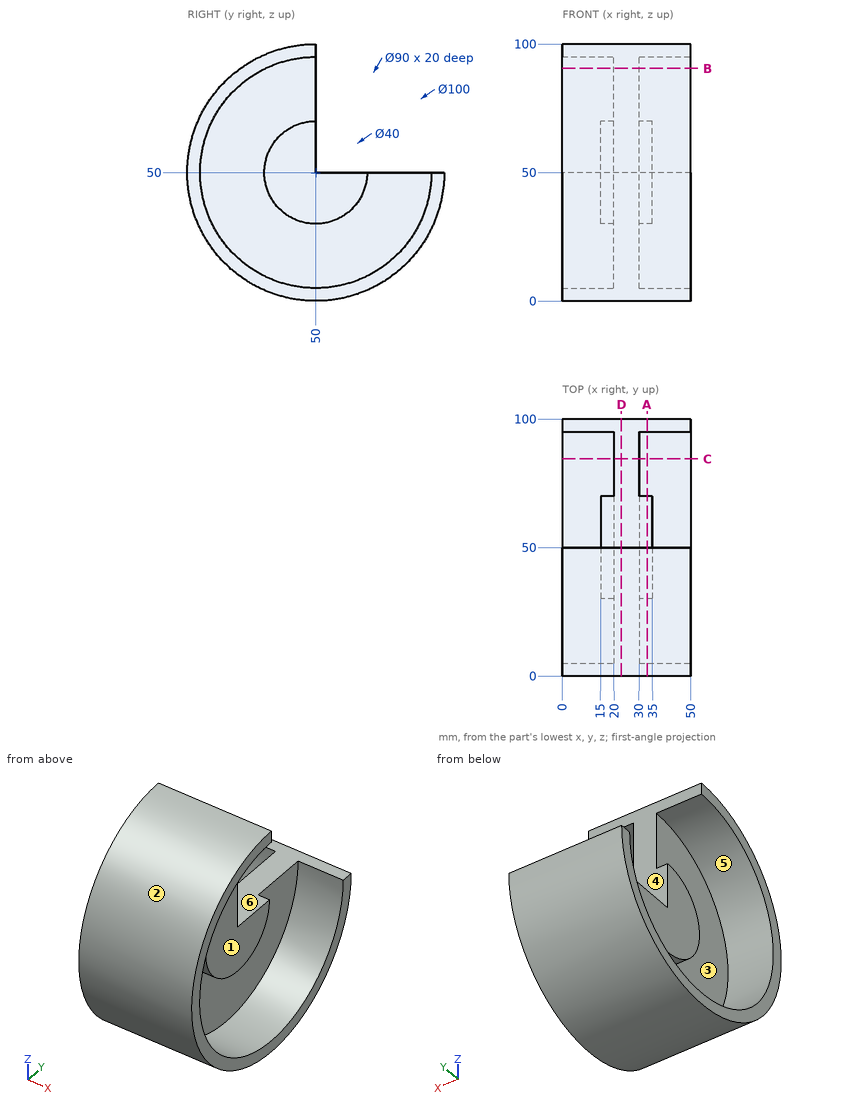
For this review, use the dimensioned drawing (mm, ordinates from the lowest corner) and the shaded views. A direction names the side the tool comes from. Give positions to 0.01 mm unless a question says otherwise; leave off trailing zeros. Loops run counter-clockwise (first coordinate to the right, second up) from the corner with the lowest first, then second, coordinate; pieces in that order, holes last. Notation, with made-up numbers: (-11, 83.5) -> (-5, 83.5) arc R22 ccw to (-5, 99.5) -> close; hole circle Ø7 at (3.5, -12). An arc over 180 degrees is marked (long way). One line per question, with ' | ' between items. Start each with the question number.
(1) Insertion check: P1, Ø1, axis at x = 20, y = 63, coming from the +Z side; P2, Ø10, axis at x = 29, z = 44.5, coming from the +Y side; P3, Ø20, axis at y = 54.5, z = 46.5, coming from the -X side. Each pin has a flat end and moves straight along its axis. Give the tip position at first contact, or say it passes through.
(2) Draft analysis for pull direction Y (two halves, no side actions). For the marked faces 4, 5 and 6, state which applies: +Y half, -Y half, draft (parallel to the pull), parting line (faces both ways), or undercut.
(3) We need section B-B (z = 90.5). State the section outline as (x, y) points, and give its area (3 significant figures).
(4) For the marked faces 1, 2 and 3, list the 3-axis set-ups (+Z, -Z, +X, -X, +Y, -Y) from which the entire face can be reached by the end or side of a thin tool; tool diameter is ignored.
(5) We need section C-C (y = 84.5). State the section outline as (x, z) points, and give its area (3 significant figures).
(6) We need section A-A (x = 33). State the section outline as (y, z) points.
(7) We need section D-D (x = 23). State the section outline as (y, z) points.
(8) For line 1 (X direction, y = 45, z = 82); line 2 (Y direction, x = 4.5, z = 13); line 3 (Y direction, x = 41, z = 16.5), list the stretches that pass through material, from the lowest coordinate up.
The answers:
1) P1: stops at z = 50 | P2: stops at y = 100 | P3: stops at x = 15
2) face 4: +Y half | face 5: undercut | face 6: draft
3) outline: (0, 20.68) -> (50, 20.68) -> (50, 30.38) -> (30, 30.38) -> (30, 50) -> (20, 50) -> (20, 30.38) -> (0, 30.38) -> close | area: 681 mm^2
4) face 1: +X | face 2: +X, -X | face 3: -X
5) outline: (0, 13.81) -> (50, 13.81) -> (50, 21.11) -> (30, 21.11) -> (30, 50) -> (20, 50) -> (20, 21.11) -> (0, 21.11) -> close | area: 654 mm^2
6) outline: (50, 50) -> (50, 70) arc R20 ccw (long way) to (70, 50) -> close; (50, 95) -> (50, 100) arc R50 ccw (long way) to (100, 50) -> (95, 50) arc R45 cw (long way) to start
7) outline: (50, 50) -> (50, 100) arc R50 ccw (long way) to (100, 50) -> close
8) line 1: x = 20 to 30 | line 2: y = 16.37 to 24.39, 75.61 to 83.63 | line 3: y = 12.88 to 19.95, 80.05 to 87.12
